Source: CAD feature listing. Evaluate the final solid. Frame: model axes, mm. Give positions to 0.01 mm unless a question says otherwise; leave off trailing zeros. Write each loop counter-clockwise with the first axis right and the second up, starting at its lowest first coordinate (ties: lowest second). Pieces come first, ordered by that corner, then holes. Notation, with made-up numbers: M 50.5,-12 L 90.5,-12 A23 ccw 90.5,15 Z; hole C -8,-38 d5. An arc over 180 degrees is marked long. Return JSON: item names as keys, results as strings.
```python
from build123d import *

# Parameters (mm, degrees)
SKETCH1_R           = 1.25
BOSS_EXTRUDE1_DEPTH = 6.35
FILLET1_R           = 0.5


with BuildPart() as part:
    # Sketch1 → Boss-Extrude1 (new body)
    with BuildSketch(Plane.XY):
        Polygon((10, 4.8), (-0.5, 4.8), (-0.5, 5.65), (-10, 5.65), (-10, -5), (10, -5), align=None)
        with Locations((-5, -2.2)):
            Circle(SKETCH1_R, mode=Mode.SUBTRACT)
        with Locations((5, -2.2)):
            Circle(SKETCH1_R, mode=Mode.SUBTRACT)
    extrude(amount=BOSS_EXTRUDE1_DEPTH)

    # Fillet1
    fillet1_edges = [part.edges().sort_by_distance(p)[0] for p in [
        (-10, 5.65, 3.175),
        (-0.5, 5.65, 3.175),
        (10, 4.8, 3.175),
        (10, -5, 3.175),
        (-10, -5, 3.175),
    ]]
    fillet(fillet1_edges, radius=FILLET1_R)


solid = part.part
```
1) Cut plane C-C, the plane z = 5. Return the cut outline in (x, y), then the cut area to 3 significant figures.
Numbers:
{"outline": "M -10,-4.5 A0.5 ccw -9.5,-5 L 9.5,-5 A0.5 ccw 10,-4.5 L 10,4.3 A0.5 ccw 9.5,4.8 L -0.5,4.8 L -0.5,5.15 A0.5 ccw -1,5.65 L -9.5,5.65 A0.5 ccw -10,5.15 Z; hole C -5,-2.2 d2.5; hole C 5,-2.2 d2.5", "area": "194 mm²"}
2) Draft query along Y for faces 1 (the face through (10, 0, 3)), 2 (the face through (0, -5, 3)), 3 (the face through (-5.99, -2.96, 3.13)), 4 (the face through (5, 4.8, 3)). Return one class per face: released by +Y, released by -Y, zero draft, split by the parting line, or undercut.
Numbers:
{"face 1": "zero draft", "face 2": "released by -Y", "face 3": "undercut", "face 4": "released by +Y"}
3) Line query: line 1 (Y direction, x = 5, z = 5); line 2 (Y direction, x = -5, z = 5.25); line 3 (X direction, y = -2.75, z = 4). Output: solid intervals per line, ascending. Write a range as [from, to].
Numbers:
{"line 1": "y = [-5, -3.45], [-0.95, 4.8]", "line 2": "y = [-5, -3.45], [-0.95, 5.65]", "line 3": "x = [-10, -6.12], [-3.88, 3.88], [6.12, 10]"}
4) Contact query for a flat-ended pin moving along its axis: pin 1 Ø1.5 at (x, y) = (-5, -2.2) entering from -Z. Output: stop coordinate, or through.
Numbers:
{"pin 1": "passes through"}
5) Cut plane A-A, the plane x = 5. Return the cut outline in (y, z), then the cut area to 3 significant figures.
Numbers:
{"outline": "M -5,0 L -3.45,0 L -3.45,6.35 L -5,6.35 Z; M -0.95,0 L 4.8,0 L 4.8,6.35 L -0.95,6.35 Z", "area": "46.4 mm²"}
6) Cut plane B-B, the plane y = -2.2. Return the cut outline in (x, z), then the cut area to 4 significant figures.
Numbers:
{"outline": "M -10,0 L -6.25,0 L -6.25,6.35 L -10,6.35 Z; M -3.75,0 L 3.75,0 L 3.75,6.35 L -3.75,6.35 Z; M 6.25,0 L 10,0 L 10,6.35 L 6.25,6.35 Z", "area": "95.25 mm²"}
7) Cut plane D-D, the plane x = -5. Return the cut outline in (y, z), then the cut area to 3 significant figures.
Numbers:
{"outline": "M -5,0 L -3.45,0 L -3.45,6.35 L -5,6.35 Z; M -0.95,0 L 5.65,0 L 5.65,6.35 L -0.95,6.35 Z", "area": "51.8 mm²"}
